Verification items for the finished model (mm, model axes). Face numbers are marked on the shaded views. Give positions to 0.01 mm unless a question says otherwise; leave off trailing zeros. Write each loop counter-clockwise with the first axis right and the second up, starting at its lowest first coordinate (ties: lowest second). Pieces come first, ordered by that corner, then holes. Notation, with made-up numbers: (-35, 25.5) -> (15, 25.5) arc R25 cw to (15, 43.5) -> close; hole circle Ø11 at (81, 15.5). An arc over 180 degrees is marked (long way). Answer as CSV lines item,"result".
```python
from build123d import *

# Parameters (mm, degrees)
PAD002_DEPTH        = 4
PAD001_DEPTH        = 3.65
PAD_DEPTH           = 43.5
CUT_PLACEMENT_ANGLE = 180


with BuildPart() as obj1:
    # Sketch002 → Pad002 (new body, symmetric)
    with BuildSketch(Plane.XZ):
        Polygon((5, 3), (13, 3), (13, -3.5), (10.19766, -6.30234), (7.80234, -6.30234), (5, -3.5), align=None)
    extrude(amount=PAD002_DEPTH, both=True)


with BuildPart() as insert001:
    # Sketch001 → Pad001 (new body, symmetric)
    with BuildSketch(Plane.XZ):
        with BuildLine():
            Line((4, -5.5), (17, -5.5))
            ThreePointArc((17, -5.5), (17.707107, -5.207107), (18, -4.5))
            Line((18, -4.5), (18, 0))
            Line((3, 0), (18, 0))
            Line((3, -4.5), (3, 0))
            ThreePointArc((3, -4.5), (3.292893, -5.207107), (4, -5.5))
        make_face()
    extrude(amount=PAD001_DEPTH, both=True)


with BuildPart() as obj2:
    # Sketch → Pad (new body, symmetric)
    with BuildSketch(Plane.XZ):
        with BuildLine():
            Line((0, 0), (18, 0))
            Line((18, 0), (18, -3))
            Line((18, -3), (19, -3))
            ThreePointArc((19, -3), (19.707107, -2.707107), (20, -2))
            Line((20, -2), (20, 1))
            ThreePointArc((20, 1), (19.707107, 1.707107), (19, 2))
            Line((19, 2), (1, 2))
            ThreePointArc((1, 2), (0.292893, 1.707107), (0, 1))
            Line((0, 1), (0, 0))
        make_face()
    extrude(amount=PAD_DEPTH, both=True)

    # Fusion: union insert001
    add(insert001.part)

    # Cut: cut obj1
    add(obj1.part, mode=Mode.SUBTRACT)


with BuildPart() as obj2_1:
    # Cut placement: moved
    add(obj2.part.moved(Location((0, 0, 2))).rotate(Axis((0, 0, 2), (1, 0, 0)), CUT_PLACEMENT_ANGLE))


solid = obj2_1.part
```
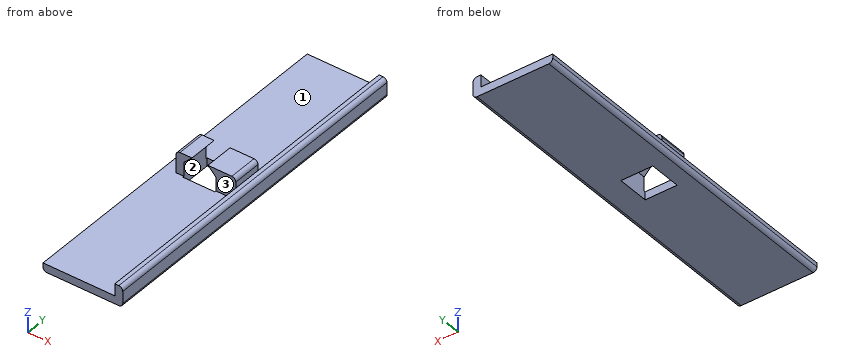
1) Section check C-C (y = -21). Record the boundary of the cut face in (x, z), and give its area (3 significant figures).
Reported:
outline,"(0, 1) arc R1 ccw to (1, 0) -> (19, 0) arc R1 ccw to (20, 1) -> (20, 4) arc R1 ccw to (19, 5) -> (18, 5) -> (18, 2) -> (0, 2) -> close"
area,"45.4 mm²"
2) Section check A-A (x = 6). Record the boundary of the cut face in (y, z).
Reported:
outline,"(-43.5, 0) -> (-4, 0) -> (-4, 2) -> (-43.5, 2) -> close; (-3.65, 6.5) -> (3.65, 6.5) -> (3.65, 7.5) -> (-3.65, 7.5) -> close; (4, 0) -> (43.5, 0) -> (43.5, 2) -> (4, 2) -> close"
3) Scan lines: line 1 along Y through (x, z) = (9, 1.25); line 2 along Y through (x, z) = (15, 2.5); line 3 along Z through (x, y) = (9.75, -13). Record each from-to range of solid material in increasing order.
Reported:
line 1,"-43.5 to -4, 4 to 43.5"
line 2,"-3.65 to 3.65"
line 3,"0 to 2"
4) Section check D-D (x = 2.25). Record the boundary of the cut face in (y, z).
Reported:
outline,"(-43.5, 0) -> (43.5, 0) -> (43.5, 2) -> (-43.5, 2) -> close"
5) Depth check by flat-ended pin: pin 1 (3 mm diameter, centred on x = 16, z = 6, fed in from +Y); pin 2 (0.5 mm diameter, centred on y = -0.5, z = 5.5, fed in from +X); pin 3 (0.9 mm diameter, centred on y = 14.5, z = 3, fed in from -X). Enter the tip coordinate at first touch or a pass-through.
Reported:
pin 1,"y = 3.65"
pin 2,"x = 18"
pin 3,"x = 18"
6) Draft check along Y on the marked faces 1, 2 and 3. Enter one of: +Y half, -Y half, draft (parallel to the pull), parting line (faces both ways), or undercut.
Reported:
face 1,"draft"
face 2,"undercut"
face 3,"-Y half"
7) Section check B-B (x = 14). Record the boundary of the cut face in (y, z), and give its area (3 significant figures).
Reported:
outline,"(-43.5, 0) -> (43.5, 0) -> (43.5, 2) -> (3.65, 2) -> (3.65, 7.5) -> (-3.65, 7.5) -> (-3.65, 2) -> (-43.5, 2) -> close"
area,"214 mm²"
